Part model, mm, in its own coordinate system. A direction names the side the tool comes from. Give positions to 0.01 mm unless a question says otherwise; leave off trailing zeros. Order: outer loops, then holes, each group sorted by start corner. A loop starts at its lowest first (then second) coordinate and runs counter-clockwise, first axis right, second up. Notation, with made-up numbers: M -37.5,20 L -27.5,20 A9 ccw -27.5,27 Z; hole C 76,-25 d7. An arc over 180 degrees is marked long. Answer as a JSON object with one key per item and string values.
from build123d import *

# Parameters (mm, degrees)
F0_W     = 76.2
F0_H     = 76.2
F1_DEPTH = 76.2
F2_W     = 12.7
F2_H     = 12.7
F3_DEPTH = 12.7
F5_DEPTH = 12.7
F7_W     = 12.7
F7_H     = 12.7
F7_W_2   = 12.64588
F8_DEPTH = 12.7


with BuildPart() as f1:
    # F0 (on Front) → F1 (new body)
    with BuildSketch(Plane.XZ):
        with Locations((-1.315733, -0.572864)):
            Rectangle(F0_W, F0_H)
    extrude(amount=F1_DEPTH)

    # F2 (on face) → F3 (cut)
    with BuildSketch(Plane.XZ.offset(76.2)):
        with Locations((30.434267, 0)):
            Rectangle(F2_W, F2_H)
    extrude(amount=-F3_DEPTH, mode=Mode.SUBTRACT)

    # F4 (on face) → F5 (cut)
    with BuildSketch(Plane.XZ.offset(76.2)):
        Polygon((6.35, -9.196139), (0, -9.196139), (-6.35, -9.196139), (-6.35, -21.642357), (6.35, -21.642357), align=None)
        Polygon((-6.35, 12.7), (0, 12.7), (6.35, 12.7), (6.35, 25.4), (-6.35, 25.4), align=None)
    extrude(amount=-F5_DEPTH, mode=Mode.SUBTRACT)

    # F7 (on face) → F8 (cut)
    with BuildSketch(Plane.YZ.offset(36.784267)):
        with Locations((-6.35, 0)):
            Rectangle(F7_W, F7_H)
        with Locations((-38.07294, -32.363346)):
            Rectangle(F7_W_2, F7_H)
        with Locations((-38.07294, 31.177136)):
            Rectangle(F7_W, F7_H)
    extrude(amount=-F8_DEPTH, mode=Mode.SUBTRACT)


solid = f1.part
1. Pin check, flat tips, straight feed: P1, Ø4, axis at x = 28.5, z = -32, coming from the +Y side; P2, Ø4, axis at x = 1, z = 18.5, coming from the -Y side; P3, Ø4, axis at x = 33.5, z = 0, coming from the +Y side; P4, Ø4, axis at x = 29, y = -39, coming from the +Z side. Stop position of each tip, or through.
Worked answers:
{"P1": "stops at y = 0", "P2": "stops at y = -63.5", "P3": "stops at y = -12.7", "P4": "stops at z = 24.83"}
2. Which spindle directions (+Z, -Z, +X, -X, +Y, -Y) get a long thin tool onto all of the face, cutting with end or side? Do faces 4 (the flat face through (0, -70, -21.642)), 5 (the flat face through (31, -12.7, 0)), 6 (the flat face through (30, -70, -6.35)), 7 (the flat face through (31, -44.423, 31)), 8 (the flat face through (31, -44.396, -32)). Say none if no direction does.
Worked answers:
{"face 4": "-Y", "face 5": "+X, +Y", "face 6": "+X, -Y", "face 7": "+Z, +X", "face 8": "-Z, +X"}
3. Probe line 1 along X through (y, z) = (-6, 6); line 2 along Y through (x, z) = (32, -5.5). List the from-to ranges inside material, lowest first.
Worked answers:
{"line 1": "x = -39.42 to 24.08", "line 2": "y = -63.5 to -12.7"}
4. Cut at D-D on y = -39. Give the cut face in (x, z).
Worked answers:
{"outline": "M -39.42,-38.67 L 24.08,-38.67 L 24.08,-26.01 L 36.78,-26.01 L 36.78,24.83 L 24.08,24.83 L 24.08,37.53 L -39.42,37.53 Z"}
5. Two-plate mould, pull along X, no slides. Class faces 1 (the flat face through (36.784, -38, -1)), 2 (the flat face through (31, -38, -26.013)), 3 (the flat face through (0, -70, 12.7)): +X half, -X half, draft (parallel to the pull), parting line (faces both ways), or undercut.
Worked answers:
{"face 1": "+X half", "face 2": "draft", "face 3": "undercut"}
6. Cut at B-B on z = 29. Give the cut face in (x, y), plus the area to 3 significant figures.
Worked answers:
{"outline": "M -39.42,-76.2 L 36.78,-76.2 L 36.78,-44.42 L 24.08,-44.42 L 24.08,-31.72 L 36.78,-31.72 L 36.78,0 L -39.42,0 Z", "area": "5,650 mm^2"}
7. Cut at A-A on y = -66.5. Give the cut face in (x, z), plus the area to 3 significant figures.
Worked answers:
{"outline": "M -39.42,-38.67 L 36.78,-38.67 L 36.78,-6.35 L 24.08,-6.35 L 24.08,6.35 L 36.78,6.35 L 36.78,37.53 L -39.42,37.53 Z; hole M -6.35,-21.64 L 6.35,-21.64 L 6.35,-9.2 L -6.35,-9.2 Z; hole M -6.35,12.7 L 6.35,12.7 L 6.35,25.4 L -6.35,25.4 Z", "area": "5,330 mm^2"}
8. Cut at C-C on x = 32.5. Give the cut face in (y, z).
Worked answers:
{"outline": "M -76.2,-38.67 L -44.4,-38.67 L -44.4,-26.01 L -31.75,-26.01 L -31.75,-38.67 L 0,-38.67 L 0,-6.35 L -12.7,-6.35 L -12.7,6.35 L 0,6.35 L 0,37.53 L -31.72,37.53 L -31.72,24.83 L -44.42,24.83 L -44.42,37.53 L -76.2,37.53 L -76.2,6.35 L -63.5,6.35 L -63.5,-6.35 L -76.2,-6.35 Z"}
